from build123d import *

# Parameters (mm, degrees)
F0_R     = 53.975
F1_DEPTH = 25.4
F2_R     = 50.8
F3_DEPTH = 19.05
F4_W     = 19.05
F4_H     = 19.05
F5_DEPTH = 12.7
F6_R     = 9.525
F7_DEPTH = 6.35
F8_W     = 17.119241
F8_H     = 19.05
F9_DEPTH = 6.35


with BuildPart() as f1:
    # F0 (on Top) → F1 (new body)
    with BuildSketch(Plane.XY):
        Circle(F0_R)
    extrude(amount=F1_DEPTH)

    # F2 (on face) → F3 (cut)
    with BuildSketch(Plane(origin=(0, 0, 0), x_dir=(1, 0, 0), z_dir=(0, 0, -1))):
        Circle(F2_R)
    extrude(amount=-F3_DEPTH, mode=Mode.SUBTRACT)

    # F4 (on face) → F5 (join)
    with BuildSketch(Plane.XY.offset(25.4)):
        Rectangle(F4_W, F4_H)
    extrude(amount=F5_DEPTH)

    # F6 (on face) → F7 (cut, through all)
    with BuildSketch(Plane.XY.offset(25.4)):
        with Locations((41.91, 0)):
            Circle(F6_R)
    extrude(amount=-F7_DEPTH, mode=Mode.SUBTRACT)

    # F8 (on face) → F9 (cut, through all)
    with BuildSketch(Plane.XY.offset(25.4)):
        with Locations((50.46962, 0)):
            Rectangle(F8_W, F8_H)
    extrude(amount=-F9_DEPTH, mode=Mode.SUBTRACT)


solid = f1.part
Build history of the part. All positions in model axes, mm. A direction names the side the tool comes from. Coordinates: 2 decimals unless noted, no trailing zeros. Write each loop counter-clockwise with the first axis right and the second up, starting at its lowest first coordinate (ties: lowest second). Pieces come first, ordered by that corner, then holes.
(1) Cut at A-A on y = 0. List the corners of the cut face in (x, z) (3 decimals), and give its area (3 significant figures).
(2) Cut at B-B on z = 8. List the corners of the cut face in (x, y) (3 decimals).
(3) Cut at C-C on x = 0. List the corners of the cut face in (y, z) (3 decimals).
(4) Cut at D-D on x = 35.5. List the corners of the cut face in (y, z).
(5) Pin check, flat tips, straight feed: pin 1 Ø3 at (x, y) = (29.5, 23) entering from -Z; pin 2 Ø10 at (x, z) = (4.5, 34) entering from -Y (3 decimals); pin 3 Ø6 at (x, z) = (15, 22.5) entering from +Y. Stop position of each tip, or through.
(6) Mould opens along X. For faces 4 (the flat face through (-1, -11, 25.4)), 5 (the flat face through (-1, -1, 19.05)), 6 (the flat face through (-9.525, 0, 32)) say: pulls with the +X half, pulls with the -X half, needs draft (parallel to the pull), parting line crosses it, or undercut.
(7) 3-axis set-ups, long thin cutter, end or side, ignore diameter. For faces 1 (the flat face through (0, 9.525, 32)), 2 (the flat face through (9.525, 0, 32)), 3 (the flat face through (52, 0, 19.05)): which of +Z, -Z, +X, -X, +Y, -Y reach the whole face in a straight line?
(8) Drill centre lines: line 1 (Y direction, x = 0, z = 5.75) (3 decimals); line 2 (Y direction, x = 17, z = 13); line 3 (Z direction, x = -36, y = -25). Where is each one in solid material? Low to high.
Working result:
1. outline: (-53.975, 0) - (-50.8, 0) - (-50.8, 19.05) - (32.385, 19.05) - (32.385, 25.4) - (9.525, 25.4) - (9.525, 38.1) - (-9.525, 38.1) - (-9.525, 25.4) - (-53.975, 25.4) - close; (50.8, 0) - (53.975, 0) - (53.975, 19.05) - (50.8, 19.05) - close
1. area: 911 mm2
2. outline: circle Ø107.95 at (0, 0); hole circle Ø101.6 at (0, 0)
3. outline: (-53.975, 0) - (-50.8, 0) - (-50.8, 19.05) - (50.8, 19.05) - (50.8, 0) - (53.975, 0) - (53.975, 25.4) - (9.525, 25.4) - (9.525, 38.1) - (-9.525, 38.1) - (-9.525, 25.4) - (-53.975, 25.4) - close
4. outline: (-40.66, 0) - (-36.34, 0) - (-36.34, 19.05) - (-7.05, 19.05) - (-7.05, 25.4) - (-40.66, 25.4) - close; (7.05, 19.05) - (36.34, 19.05) - (36.34, 0) - (40.66, 0) - (40.66, 25.4) - (7.05, 25.4) - close
5. pin 1: stops at z = 19.05
5. pin 2: stops at y = -9.525
5. pin 3: stops at y = 52.62
6. face 4: needs draft
6. face 5: undercut
6. face 6: pulls with the -X half
7. face 1: +Z, +X, -X, +Y
7. face 2: +Z, +X, +Y, -Y
7. face 3: +Z, +X
8. line 1: y = -53.975 to -50.8, 50.8 to 53.975
8. line 2: y = -51.23 to -47.87, 47.87 to 51.23
8. line 3: z = 19.05 to 25.4
